Verification items for the finished model (mm, model axes). A direction names the side the tool comes from. Give positions to 0.01 mm unless a question says otherwise; leave off trailing zeros. Write each loop counter-clockwise with the first axis right and the second up, starting at its lowest first coordinate (ties: lowest second). Pieces come first, ordered by that corner, then holes.
from build123d import *

# Parameters (mm, degrees)
BASE_R              = 27.5
BASE_R_2            = 10.425
BASE_R_3            = 6.425
BASE_R_4            = 8.275
BOSS_EXTRUDE1_DEPTH = 3.25
BASE_4_R            = 8.275
BASE_4_R_2          = 6.425
BOSS_EXTRUDE2_DEPTH = 16
BASE_5_R            = 10.425
BASE_5_R_2          = 8.275
BOSS_EXTRUDE3_DEPTH = 12


with BuildPart() as part:
    # Base → Boss-Extrude1 (new body)
    with BuildSketch(Plane(origin=(0, 0, 0), x_dir=(1, 0, 0), z_dir=(0, 1, 0))):
        Circle(BASE_R)
        Circle(BASE_R_2, mode=Mode.SUBTRACT)
        Circle(BASE_R_2)
        Circle(BASE_R_3, mode=Mode.SUBTRACT)
        Circle(BASE_R_4)
        Circle(BASE_R_3, mode=Mode.SUBTRACT)
    extrude(amount=BOSS_EXTRUDE1_DEPTH)

    # Base_4 → Boss-Extrude2 (add)
    with BuildSketch(Plane(origin=(0, 0, 0), x_dir=(1, 0, 0), z_dir=(0, 1, 0))):
        Circle(BASE_4_R)
        Circle(BASE_4_R_2, mode=Mode.SUBTRACT)
    extrude(amount=BOSS_EXTRUDE2_DEPTH)

    # Base_5 → Boss-Extrude3 (add)
    with BuildSketch(Plane(origin=(0, 0, 0), x_dir=(1, 0, 0), z_dir=(0, 1, 0))):
        Circle(BASE_5_R)
        Circle(BASE_5_R_2, mode=Mode.SUBTRACT)
    extrude(amount=BOSS_EXTRUDE3_DEPTH)


solid = part.part
Item 1: Depth check by flat-ended pin: pin 1 (8 mm diameter, centred on x = 11.5, z = 19.5, fed in from +Y); pin 2 (1.5 mm diameter, centred on y = 11, z = -6.5, fed in from -X). Enter the tip coordinate at first touch or a pass-through.
Answer key:
pin 1: stops at y = 3.25
pin 2: stops at x = -8.7
Item 2: Sectioned sample at D-D on z = 17. Record the cut outline in (x, y).
Answer key:
outline: (-21.62, 0) - (21.62, 0) - (21.62, 3.25) - (-21.62, 3.25) - close
Item 3: Scan lines: line 1 along X through (y, z) = (4.25, 0) (3 decimals); line 2 along Z through (x, y) = (0, 12.5) (3 decimals). Record each from-to range of solid material in increasing order.
Answer key:
line 1: x = -10.425 to -6.425, 6.425 to 10.425
line 2: z = -8.275 to -6.425, 6.425 to 8.275
Item 4: Sectioned sample at B-B on z = 0. Record the cut outline in (x, y) (3 decimals), then the cut area to 3 significant figures.
Answer key:
outline: (-27.5, 0) - (-6.425, 0) - (-6.425, 16) - (-8.275, 16) - (-8.275, 12) - (-10.425, 12) - (-10.425, 3.25) - (-27.5, 3.25) - close; (6.425, 0) - (27.5, 0) - (27.5, 3.25) - (10.425, 3.25) - (10.425, 12) - (8.275, 12) - (8.275, 16) - (6.425, 16) - close
area: 222 mm2
Item 5: Release check for a two-part mould opening along X. For faces 1 (the face through (-1.357, 7.564, -10.336)), 2 (the face through (-5.1, 7.89, 3.91)), 3 (the face through (-3, 12, -8)) record: released by +X, released by -X, zero draft, split by the parting line, or undercut.
Answer key:
face 1: split by the parting line
face 2: undercut
face 3: zero draft
Item 6: Set-up check for faces 4 (the face through (6, 0, 6)), 5 (the face through (-1.79, 13.97, 8.08)): record each of +Z, -Z, +X, -X, +Y, -Y from which the full face is reachable in a straight line by a thin tool's end or side.
Answer key:
face 4: +Z, -Z, +X, -X, -Y
face 5: +Y
Item 7: Sectioned sample at C-C on y = 7. Record the cut outline in (x, z) (3 decimals), then the cut area to 3 significant figures.
Answer key:
outline: circle Ø20.85 at (0, 0); hole circle Ø12.85 at (0, 0)
area: 212 mm2
Item 8: Sectioned sample at A-A on x = 0. Record the cut outline in (y, z) (3 decimals).
Answer key:
outline: (0, -27.5) - (3.25, -27.5) - (3.25, -10.425) - (12, -10.425) - (12, -8.275) - (16, -8.275) - (16, -6.425) - (0, -6.425) - close; (0, 6.425) - (16, 6.425) - (16, 8.275) - (12, 8.275) - (12, 10.425) - (3.25, 10.425) - (3.25, 27.5) - (0, 27.5) - close
